from build123d import *

# Parameters (mm, degrees)
F0_W      = 25
F0_H      = 100
F1_DEPTH  = 300
F3_DEPTH  = 80
F5_DEPTH  = 80
F7_DEPTH  = 15
F9_DEPTH  = 15
F11_DEPTH = 15
F13_DEPTH = 15
F15_DEPTH = 15
F17_DEPTH = 15
F19_DEPTH = 15
F21_DEPTH = 15
F23_DEPTH = 300
F24_W     = 7.5
F24_H     = 60
F25_DEPTH = 10
F26_W     = 2.5
F26_H     = 15
F27_DEPTH = 20
F28_W     = 10
F28_H     = 15
F29_DEPTH = 2.5


# Not quite as in the source:
# - a pattern or mirror of a feature is missing from the dataset's text; its kind, count and spacing are read off the source's solid


with BuildPart() as f1:
    # F0 (on Front) → F1 (new body)
    with BuildSketch(Plane.XZ):
        Rectangle(F0_W, F0_H)
    extrude(amount=F1_DEPTH)

    # F2 (on face) → F3 (cut)
    with BuildSketch(Plane.YZ.offset(12.5)):
        Polygon((-180, 20), (-120, 20), (0, 50), (-300, 50), align=None)
    extrude(amount=-F3_DEPTH, mode=Mode.SUBTRACT)

    # F4 (on face) → F5 (cut)
    with BuildSketch(Plane(origin=(-12.5, 0, 0), x_dir=(0, -1, 0), z_dir=(-1, 0, 0))):
        Polygon((180, -20), (120, -20), (0, -50), (300, -50), align=None)
    extrude(amount=-F5_DEPTH, mode=Mode.SUBTRACT)

    # F6 (on face) → F7 (cut)
    with BuildSketch(Plane.XZ.offset(300)):
        with BuildLine():
            Line((-12.5, 45), (-12.5, -45))
            ThreePointArc((-12.5, -45), (5.5958424018, 0), (-12.5, 45))
        make_face()
    f7 = extrude(amount=-F7_DEPTH, mode=Mode.SUBTRACT)

    # F7_copies: F7 across plane
    add(f7.mirror(Plane.ZX.offset(-150)), mode=Mode.SUBTRACT)

    # F8 (on face) → F9 (cut)
    with BuildSketch(Plane.XZ.offset(285)):
        with BuildLine():
            Line((-12.5, 40), (-12.5, -40))
            ThreePointArc((-12.5, -40), (2.77864045, 0), (-12.5, 40))
        make_face()
    f9 = extrude(amount=-F9_DEPTH, mode=Mode.SUBTRACT)

    # F9_copies: F9 across plane
    add(f9.mirror(Plane.ZX.offset(-150)), mode=Mode.SUBTRACT)

    # F10 (on face) → F11 (cut)
    with BuildSketch(Plane.XZ.offset(270)):
        with BuildLine():
            Line((-12.5, 35), (-12.5, -35))
            ThreePointArc((-12.5, -35), (-1.233971724, 0), (-12.5, 35))
        make_face()
    f11 = extrude(amount=-F11_DEPTH, mode=Mode.SUBTRACT)

    # F11_copies: F11 across plane
    add(f11.mirror(Plane.ZX.offset(-150)), mode=Mode.SUBTRACT)

    # F12 (on face) → F13 (cut)
    with BuildSketch(Plane.XZ.offset(255)):
        with BuildLine():
            Line((-12.5, 30), (-12.5, -30))
            ThreePointArc((-12.5, -30), (-4.4615242271, 0), (-12.5, 30))
        make_face()
    f13 = extrude(amount=-F13_DEPTH, mode=Mode.SUBTRACT)

    # F13_copies: F13 across plane
    add(f13.mirror(Plane.ZX.offset(-150)), mode=Mode.SUBTRACT)

    # F14 (on face) → F15 (cut)
    with BuildSketch(Plane.XZ.offset(240)):
        with BuildLine():
            Line((-12.5, 25), (-12.5, -25))
            ThreePointArc((-12.5, -25), (-7.0435605732, 0), (-12.5, 25))
        make_face()
    f15 = extrude(amount=-F15_DEPTH, mode=Mode.SUBTRACT)

    # F15_copies: F15 across plane
    add(f15.mirror(Plane.ZX.offset(-150)), mode=Mode.SUBTRACT)

    # F16 (on face) → F17 (cut)
    with BuildSketch(Plane.XZ.offset(225)):
        with BuildLine():
            Line((-12.5, 20), (-12.5, -20))
            ThreePointArc((-12.5, -20), (-9.0685424949, 0), (-12.5, 20))
        make_face()
    f17 = extrude(amount=-F17_DEPTH, mode=Mode.SUBTRACT)

    # F17_copies: F17 across plane
    add(f17.mirror(Plane.ZX.offset(-150)), mode=Mode.SUBTRACT)

    # F18 (on face) → F19 (cut)
    with BuildSketch(Plane.XZ.offset(210)):
        with BuildLine():
            Line((-12.5, 15), (-12.5, -15))
            ThreePointArc((-12.5, -15), (-10.5947501931, 0), (-12.5, 15))
        make_face()
    f19 = extrude(amount=-F19_DEPTH, mode=Mode.SUBTRACT)

    # F19_copies: F19 across plane
    add(f19.mirror(Plane.ZX.offset(-150)), mode=Mode.SUBTRACT)

    # F20 (on face) → F21 (cut)
    with BuildSketch(Plane.XZ.offset(195)):
        with BuildLine():
            Line((-12.5, 10), (-12.5, -10))
            ThreePointArc((-12.5, -10), (-11.660797831, 0), (-12.5, 10))
        make_face()
    f21 = extrude(amount=-F21_DEPTH, mode=Mode.SUBTRACT)

    # F21_copies: F21 across plane
    add(f21.mirror(Plane.ZX.offset(-150)), mode=Mode.SUBTRACT)

    # F22 (on face) → F23 (cut)
    with BuildSketch(Plane.XZ.offset(300)):
        with BuildLine():
            Line((12.5, 50), (-12.5, 50))
            ThreePointArc((-12.5, 50), (8.5102051443, 0), (-12.5, -50))
            Line((-12.5, -50), (12.5, -50))
            Line((12.5, -50), (12.5, 50))
        make_face()
    extrude(amount=-F23_DEPTH, mode=Mode.SUBTRACT)

    # F24 (on face) → F25 (cut)
    with BuildSketch(Plane.XY.offset(20)):
        with Locations((-8.75, -150)):
            Rectangle(F24_W, F24_H)
    extrude(amount=-F25_DEPTH, mode=Mode.SUBTRACT)

    # F26 (on face) → F27 (cut)
    with BuildSketch(Plane.XY.offset(10)):
        with Locations((-11.25, -162.5)):
            Rectangle(F26_W, F26_H)
        with Locations((-11.25, -137.5)):
            Rectangle(F26_W, F26_H)
    extrude(amount=-F27_DEPTH, mode=Mode.SUBTRACT)

    # F28 (on face) → F29 (cut)
    with BuildSketch(Plane(origin=(-12.5, 0, 0), x_dir=(0, -1, 0), z_dir=(-1, 0, 0))):
        with Locations((175, -2.5)):
            Rectangle(F28_W, F28_H)
    extrude(amount=-F29_DEPTH, mode=Mode.SUBTRACT)


solid = f1.part
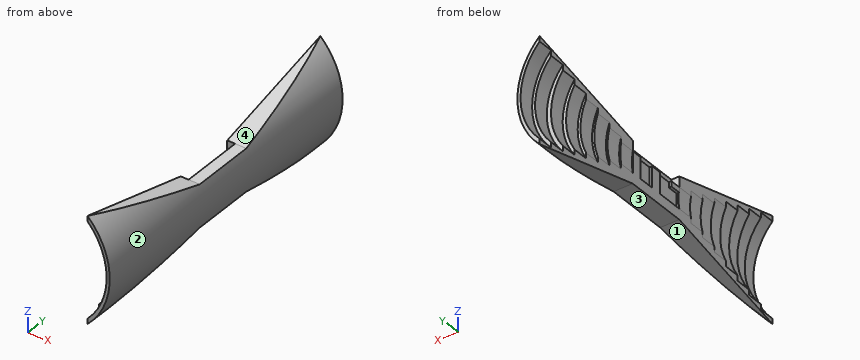
Verification items for the finished model (mm, model axes). Face numbers are marked on the shaded views. A direction names the side the tool comes from. Give positions to 0.01 mm unless a question says otherwise; leave off trailing zeros. Write each loop counter-clockwise with the first axis right and the second up, starting at its lowest first coordinate (ties: lowest second). Pieces come first, ordered by that corner, then holes.
(1) Cross-section at B-B (y = -280.5). Enter the section's corners in (x, z) (3 decimals).
(2) Access from +Z, -Z, +X, -X, +Y, -Y to the whole of each face (thin tool, end or side, straight path). Record for the marked faces 1 and 2.
(3) Gauge pin test, flat ends, axial feed: pin 1 (10 mm diameter, centred on y = -165.5, z = -3.5, fed in from -X); pin 2 (4 mm diameter, centred on x = -6.5, z = -6.5, fed in from +Y); pin 3 (8 mm diameter, centred on x = 5.5, y = -92.5, fed in from +Z). Record the tip position at first contact, or that the pin passes through.
(4) Cross-section at A-A (y = -51). Enter the section's corners in (x, z).
(5) Mould release check, pull along Y, two halves, no side actions. Record for the marked faces 3 and 4: +Y half, -Y half, draft (parallel to the pull), parting line (faces both ways), or undercut.
(6) Material ranges on line 1 (Z direction, x = -2.5, y = -127.5); line 2 (Z direction, x = -11.25, y = -241); line 3 (Y direction, x = -8, z = 15), recorded low to high.
Worked out:
1. outline: (-12.5, -45.125) - (-7.976, -45.125) arc R70 ccw to (-7.976, 45.125) - (-12.5, 45.125) - (-12.5, 40) arc R60 cw to (-12.5, -40) - close
2. face 1: -Z, +X, -X
2. face 2: +X, +Y, -Y
3. pin 1: stops at x = -10
3. pin 2: stops at y = -45
3. pin 3: stops at z = 27.62
4. outline: (-12.5, -37.25) - (-2.22, -37.25) arc R70 ccw to (-2.22, 37.25) - (-12.5, 37.25) - (-12.5, 30) arc R60 cw to (-12.5, -30) - close
5. face 3: undercut
5. face 4: undercut
6. line 1: z = -20 to 20
6. line 2: z = -35.25 to -27.72, 27.72 to 35.25
6. line 3: y = -240 to -180, -120 to -60
